Geometry: final body of the model. Coordinates: model frame, mm. A direction names the side the tool comes from. Round coordinates to 2 decimals unless told otherwise and drop trailing zeros. Write each loop counter-clockwise with the first axis right and the second up, starting at its lowest first coordinate (ties: lowest second). Pieces come first, ordered by that corner, then holes. Notation, with made-up numbers: (48, 73) - (66, 73) arc R30 cw to (66, 99) - close; hole circle Ø7 at (52, 85). An arc over 180 degrees is marked (long way). Write each question's results on one line, items separated by ' | '.
from build123d import *

# Parameters (mm, degrees)
BOSS_EXTRUDE1_DEPTH = 20
SKETCH2_R           = 4
BOSS_EXTRUDE2_DEPTH = 20
BOSS_EXTRUDE3_DEPTH = 2
BOSS_EXTRUDE4_DEPTH = 18
CUT_EXTRUDE1_DEPTH  = 22
BOSS_EXTRUDE5_DEPTH = 2
SKETCH8_R           = 2
CUT_EXTRUDE3_DEPTH  = 0.7
CUT_EXTRUDE2_REACH  = 94.752
SKETCH6_W           = 19.696996452
SKETCH6_H           = 13.58493718
CUT_EXTRUDE4_REACH  = 94.752
BOSS_EXTRUDE6_START = -2
BOSS_EXTRUDE6_DEPTH = 2
BOSS_EXTRUDE7_DEPTH = 2
BOSS_EXTRUDE8_START = -20
BOSS_EXTRUDE8_DEPTH = 20


with BuildPart() as part:
    # Sketch1 → Boss-Extrude1 (new body)
    with BuildSketch(Plane(origin=(0, 0, 0), x_dir=(1, 0, 0), z_dir=(0, 1, 0))):
        with BuildLine():
            Line((0, -15.5), (0, -63))
            Line((0, -63), (-14, -63))
            Line((-14, -63), (-14, -12.093386622))
            ThreePointArc((-14, -12.093386622), (-16.822271733, 7.698127938), (0, 18.5))
            Line((0, 18.5), (0, 15.5))
            ThreePointArc((0, 15.5), (-15.5, 0), (0, -15.5))
        make_face()
        with BuildLine():
            Line((-11, -60), (-11, -14.874474781))
            ThreePointArc((-11, -14.874474781), (-7.201195596, -17.04091494), (-3, -18.255136264))
            Line((-3, -18.255136264), (-3, -60))
            Line((-3, -60), (-11, -60))
        make_face(mode=Mode.SUBTRACT)
    extrude(amount=BOSS_EXTRUDE1_DEPTH)

    # Sketch2 → Boss-Extrude2 (add)
    with BuildSketch(Plane.XY.offset(63)):
        with Locations(Location((-7, 10, 0), (0, 0, 180))):
            Circle(SKETCH2_R)
    extrude(amount=BOSS_EXTRUDE2_DEPTH)

    # Sketch3 → Boss-Extrude3 (add)
    with BuildSketch(Plane(origin=(0, 20, 0), x_dir=(1, 0, 0), z_dir=(0, 1, 0))):
        with BuildLine():
            Line((0, -63), (10.749394376, -63))
            Line((10.749394376, -63), (10.749394376, -76))
            Line((10.749394376, -76), (13.249394376, -76))
            Line((13.249394376, -76), (13.249394376, -73))
            ThreePointArc((13.249394376, -73), (14.249394376, -72), (15.249394376, -73))
            Line((15.249394376, -73), (15.249394376, -76))
            Line((15.249394376, -76), (17.749394376, -76))
            Line((17.749394376, -76), (17.749394376, -56))
            Line((17.749394376, -56), (0, -56))
            Line((0, -56), (0, -63))
        make_face()
        Polygon((2, -58), (15.749394376, -58), (15.749394376, -69), (12.749394376, -69), (12.749394376, -61), (2, -61), align=None, mode=Mode.SUBTRACT)
    extrude(amount=-BOSS_EXTRUDE3_DEPTH)

    # Sketch4 → Boss-Extrude4 (add)
    with BuildSketch(Plane.XZ.offset(-18)):
        Polygon((15.749394376, 69), (15.749394376, 58), (2, 58), (2, 61), (12.749394376, 61), (12.749394376, 69), (12.749394376, 76), (10.749394376, 76), (10.749394376, 66), (10.749394376, 63), (0, 63), (0, 56), (17.749394376, 56), (17.749394376, 66), (17.749394376, 76), (15.749394376, 76), align=None)
    extrude(amount=BOSS_EXTRUDE4_DEPTH)

    # Sketch5 → Cut-Extrude1 (cut)
    with BuildSketch(Plane(origin=(0, 0, 56), x_dir=(-1, 0, 0), z_dir=(0, 0, -1))):
        Polygon((0, 0), (-17.749394376, 14), (-17.749394376, -1.554529852), (0, -1.554529852), align=None)
    extrude(amount=-CUT_EXTRUDE1_DEPTH, mode=Mode.SUBTRACT)

    # Sketch7 → Boss-Extrude5 (add)
    with BuildSketch(Plane(origin=(0, 20, 0), x_dir=(1, 0, 0), z_dir=(0, 1, 0))):
        Polygon((2, -61), (12.749394376, -61), (12.749394376, -69), (15.749394376, -69), (15.749394376, -58), (2, -58), align=None)
    extrude(amount=-BOSS_EXTRUDE5_DEPTH)

    # Sketch8 → Cut-Extrude3 (cut)
    with BuildSketch(Plane(origin=(0, 20, 0), x_dir=(1, 0, 0), z_dir=(0, 1, 0))):
        with Locations((14.249394376, -73)):
            Circle(SKETCH8_R)
    extrude(amount=-CUT_EXTRUDE3_DEPTH, mode=Mode.SUBTRACT)

    # Cut-Extrude2: up to this face of the body (flat: up to its plane)
    cut_extrude2_end = Plane(part.part.faces().sort_by_distance((10.749394376, 14.239342427, 69.5))[0])
    # Sketch6 → Cut-Extrude2 (cut, up to the picked face)
    with BuildSketch(Plane(origin=(17.749394376, 0, 0), x_dir=(0, 0, -1), z_dir=(1, 0, 0)), mode=Mode.PRIVATE) as cut_extrude2_sk1:
        with Locations((-72.848498226, 7.20753141)):
            Rectangle(SKETCH6_W, SKETCH6_H)
    cut_extrude2_tool1 = split(extrude(cut_extrude2_sk1.sketch, amount=-CUT_EXTRUDE2_REACH, mode=Mode.PRIVATE), bisect_by=cut_extrude2_end, keep=Keep.BOTH, mode=Mode.PRIVATE)
    add(cut_extrude2_tool1.solids().sort_by(Axis((17.749394, 7.207531, 72.848498), (-1, 0, 0)))[0], mode=Mode.SUBTRACT)

    # Cut-Extrude4: up to this face of the body (flat: up to its plane)
    cut_extrude4_end = Plane(part.part.faces().sort_by_distance((10.749394376, 17, 69.5))[0])
    # Sketch10 → Cut-Extrude4 (cut, up to the picked face)
    with BuildSketch(Plane(origin=(17.749394376, 0, 0), x_dir=(0, 0, -1), z_dir=(1, 0, 0)), mode=Mode.PRIVATE) as cut_extrude4_sk1:
        Polygon((-63, 14), (-76, 18), (-76, 12.216867542), (-63, 12.216867542), align=None)
    cut_extrude4_tool1 = split(extrude(cut_extrude4_sk1.sketch, amount=-CUT_EXTRUDE4_REACH, mode=Mode.PRIVATE), bisect_by=cut_extrude4_end, keep=Keep.BOTH, mode=Mode.PRIVATE)
    add(cut_extrude4_tool1.solids().sort_by(Axis((17.749394, 14.284655, 70.645435), (-1, 0, 0)))[0], mode=Mode.SUBTRACT)

    # Sketch11 → Boss-Extrude6 (add)
    with BuildSketch(Plane(origin=(0, 20, 0), x_dir=(1, 0, 0), z_dir=(0, 1, 0)).offset(BOSS_EXTRUDE6_START)):
        with BuildLine():
            Line((-11, -14.874474781), (-11, -60))
            Line((-11, -60), (-3, -60))
            Line((-3, -60), (-3, -18.255136264))
            ThreePointArc((-3, -18.255136264), (-7.201195596, -17.04091494), (-11, -14.874474781))
        make_face()
    extrude(amount=BOSS_EXTRUDE6_DEPTH)

    # Sketch12 → Boss-Extrude7 (add)
    with BuildSketch(Plane.XZ):
        with BuildLine():
            Line((-3, 60), (-3, 18.255136264))
            ThreePointArc((-3, 18.255136264), (-7.201195596, 17.04091494), (-11, 14.874474781))
            Line((-11, 14.874474781), (-11, 60))
            Line((-11, 60), (-3, 60))
        make_face()
    extrude(amount=-BOSS_EXTRUDE7_DEPTH)

    # Sketch13 → Boss-Extrude8 (add)
    with BuildSketch(Plane(origin=(0, 20, 0), x_dir=(1, 0, 0), z_dir=(0, 1, 0)).offset(BOSS_EXTRUDE8_START)):
        with BuildLine():
            Line((0, 15.5), (0, 18.5))
            ThreePointArc((0, 18.5), (18.390272559, 2.011933204), (4, -18.062391868))
            Line((4, -18.062391868), (4, -35))
            Line((4, -35), (0.01, -35))
            Line((0.01, -35), (0.01, -15.499996774))
            ThreePointArc((0.01, -15.499996774), (15.499999194, 0.005), (0, 15.5))
        make_face()
    extrude(amount=BOSS_EXTRUDE8_DEPTH)


solid = part.part
Q1. Ray query, line 1 along X through (y, z) = (19.8, 73); line 2 along X through (y, z) = (12, 46); line 3 along Y through (x, z) = (-6, 39). Return the intervals inside material, ascending.
Answer block:
line 1: 10.75 to 12.25, 16.25 to 17.75 | line 2: -14 to -11, -3 to 0 | line 3: 0 to 2, 18 to 20
Q2. Section query C-C, the plane x = -12. Return loops of the section in (y, z).
Answer block:
outline: (0, -14.08) - (20, -14.08) - (20, -9.81) - (0, -9.81) - close; (0, 9.81) - (20, 9.81) - (20, 63) - (0, 63) - close
Q3. Section query A-A, the plane x = -7. Return loops of the section in (y, z), plus the area to 3 significant figures.
Answer block:
outline: (0, -17.12) - (20, -17.12) - (20, -13.83) - (0, -13.83) - close; (0, 13.83) - (20, 13.83) - (20, 63) - (14, 63) - (14, 83) - (6, 83) - (6, 63) - (0, 63) - close; hole (2, 17.12) - (18, 17.12) - (18, 60) - (2, 60) - close | area: 523 mm2
Q4. Pin query (flat end, axial travel): pin 1 (12 mm diameter, centred on y = 4.5, z = 63.5, fed in from -X); pin 2 (1.5 mm diameter, centred on x = -9.5, y = 8, fed in from -Z); pin 3 (4 mm diameter, centred on y = 6, z = 36.5, fed in from +X). Return the tip coordinate at first contact, or that it passes through.
Answer block:
pin 1: x = -14 | pin 2: z = -16.3 | pin 3: x = 4
Q5. Section query B-B, the plane z = 0. Return loops of the section in (x, y).
Answer block:
outline: (-18.5, 0) - (-15.5, 0) - (-15.5, 20) - (-18.5, 20) - close; (15.5, 0) - (18.5, 0) - (18.5, 20) - (15.5, 20) - close
Q6. Mould query, pull axis Y, two halves, no side actions, for faces 6 (the cylindrical face through (14.3, 19.7, 71)), 7 (the flat face through (11.763, 15.972, 69.409)), 8 (the flat face through (-7, 2, 38)). Classes: pulls with the +Y half, pulls with the -Y half, needs draft (parallel to the pull), parting line crosses it, or undercut.
Answer block:
face 6: needs draft | face 7: pulls with the -Y half | face 8: undercut
Q7. Access query for faces 1 (the flat face through (-7, 18, 37)), 2 (the flat face through (17.749, 18, 64)), 3 (the flat face through (7, 12, 56)), 4 (the flat face through (12.749, 15, 65)), 5 (the flat face through (13.249, 19, 75)). Directions: +Z, -Z, +X, -X, +Y, -Y. A direction counts if a zero-diameter tool reaches every point of the face in a straight line with its end or side. Return the directions, or none.
Answer block:
face 1: none | face 2: +Z, +X, +Y, -Y | face 3: +X, +Y, -Y | face 4: +Z, -Y | face 5: +Z, +Y, -Y
